Autodesk Inventor part; units mm, degrees
ref_plane "YZ Plane" through (0, 0, 0) normal (1, 0, 0) x (0, 1, 0)
ref_plane "XZ Plane" through (0, 0, 0) normal (0, 1, 0) x (-1, 0, 0)
ref_plane "XY Plane" through (0, 0, 0) normal (0, 0, 1) x (1, 0, 0)
sketch "Sketch1" plane through (0, 0, 0) normal (0, 1, 0) x (-1, 0, 0)
  line L0 (0, 0) -> (10, 0)
  line L1 (10, 0) -> (66.654, -9.9896)
  line L2 (66.654, -9.9896) -> (66.654, -41.5096)
  line L3 (66.654, -41.5096) -> (2, -133.8451)
  line L4 (2, -133.8451) -> (0, -133.8451)
  line L5 (0, -133.8451) -> (0, 0)
  dimension "d0" = 31.52
  dimension "d1" = 145
  dimension "d2" = 100
  dimension "d3" = 10
  dimension "d4" = 2
  dimension "d5" = 66.654
extrude "Extrusion1" add sketch "Sketch1" along normal blind 6.5
sketch "Sketch2" plane through (0, 6.5, 0) normal (0, 1, 0) x (1, 0, 0)
  line L0 (-66.654, 41.5096) -> (-66.654, 9.9896)
  line L1 (-66.654, 9.9896) -> (-10, 0)
  line L2 (-50.354, 26.3816) -> (-50.354, 21.8816)
  line L3 (-66.654, 21.8816) -> (-66.654, 26.3816)
  line L4 (-61.654, 28.8816) -> (-54.354, 28.8816)
  line L5 (-54.354, 19.3816) -> (-61.654, 19.3816)
  line L6 (-66.654, 26.3816) -> (-61.654, 26.3816)
  line L7 (-54.354, 26.3816) -> (-50.354, 26.3816)
  line L8 (-61.654, 19.3816) -> (-61.654, 21.8816)
  line L9 (-61.654, 26.3816) -> (-61.654, 28.8816)
  line L10 (-50.354, 21.8816) -> (-54.354, 21.8816)
  line L11 (-61.654, 21.8816) -> (-66.654, 21.8816)
  line L12 (-54.354, 28.8816) -> (-54.354, 26.3816)
  line L13 (-54.354, 21.8816) -> (-54.354, 19.3816)
  line L14 (-37.7124, 21.4379) -> (-33.2807, 20.6565)
  line L15 (-36.1112, 4.6041) -> (-40.5428, 5.3855)
  line L16 (-42.1366, 10.7437) -> (-40.869, 17.9328)
  line L17 (-31.5133, 16.2831) -> (-32.7809, 9.094)
  line L18 (-40.5428, 5.3855) -> (-39.6746, 10.3096)
  line L19 (-38.4069, 17.4987) -> (-37.7124, 21.4379)
  line L20 (-32.7809, 9.094) -> (-35.2429, 9.5281)
  line L21 (-39.6746, 10.3096) -> (-42.1366, 10.7437)
  line L22 (-33.2807, 20.6565) -> (-33.9753, 16.7172)
  line L23 (-35.2429, 9.5281) -> (-36.1112, 4.6041)
  line L24 (-40.869, 17.9328) -> (-38.4069, 17.4987)
  line L25 (-33.9753, 16.7172) -> (-31.5133, 16.2831)
  point P0 (-38.327, 4.9948)
  point P1 (-50.354, 24.1316)
  dimension "d8" = 4.5
  dimension "d9" = 5
  dimension "d10" = 4
  dimension "d11" = 7.3
  dimension "d12" = 2.5
  dimension "d13" = 4.5
  dimension "d14" = 5
  dimension "d15" = 4
  dimension "d16" = 7.3
  dimension "d17" = 2.5
  dimension "d35" = 14.142
extrude "Extrusion2" cut sketch "Sketch2" against normal through all
sketch "Sketch3" plane through (0, 6.5, 0) normal (0, 1, 0) x (1, 0, 0)
  line L0 (-66.654, 9.9896) -> (-40.5428, 5.3855)
  line L1 (-37.7124, 21.4379) -> (-33.2807, 20.6565)
  line L2 (-36.1112, 4.6041) -> (-10, 0)
  line L3 (-45.7131, 6.2972) -> (-53.5915, 7.6864)
  line L4 (-53.5915, 7.6864) -> (-54.3729, 3.2547)
  line L5 (-52.7506, 0.9378) -> (-48.8114, 0.2432)
  line L6 (-46.4945, 1.8655) -> (-45.7131, 6.2972)
  line L7 (-30.9409, 3.6925) -> (-23.0625, 2.3033)
  line L8 (-23.0625, 2.3033) -> (-23.8439, -2.1284)
  line L9 (-26.1608, -3.7507) -> (-30.1, -3.0561)
  line L10 (-31.7224, -0.7392) -> (-30.9409, 3.6925)
  arc A0 (-54.3729, 3.2547) -> (-52.7506, 0.9378) centre (-52.4033, 2.9074) ccw
  arc A1 (-48.8114, 0.2432) -> (-46.4945, 1.8655) centre (-48.4641, 2.2128) ccw
  arc A2 (-31.7224, -0.7392) -> (-30.1, -3.0561) centre (-29.7527, -1.0865) ccw
  arc A3 (-26.1608, -3.7507) -> (-23.8439, -2.1284) centre (-25.8135, -1.7811) ccw
  point P0 (-35.4965, 21.0472)
  dimension "d20" = 2
  dimension "d21" = 8
  dimension "d22" = 8
  dimension "d23" = 6.5
  dimension "d24" = 15
  dimension "d25" = 7.5
extrude "Extrusion3" add sketch "Sketch3" against normal blind 6.5
sketch "Sketch4" plane through (0, 6.5, 0) normal (0, 1, 0) x (1, 0, 0)
  line L0 (-23.0625, 2.3033) -> (-10, 0)
  line L1 (-10, 0) -> (0, 0)
  line L2 (0, 0) -> (0, 133.8451)
  line L3 (-61.654, 19.3816) -> (-61.654, 21.8816)
  line L4 (0, 50) -> (-10, 50)
  line L5 (-10, 50) -> (-14, 46)
  line L6 (-14, 46) -> (-14, 0.7053)
  dimension "d28" = 45
  dimension "d29" = 10
  dimension "d30" = 50
  dimension "d32" = 4
extrude "Extrusion4" cut sketch "Sketch4" against normal through all
sketch "Sketch5" plane through (0, 6.5, 0) normal (0, 1, 0) x (1, 0, 0)
  line L0 (0, 50) -> (0, 133.8451)
  line L1 (0, 62.001) -> (4.5, 62.001)
  line L2 (6.5, 64.001) -> (6.5, 68.001)
  line L3 (4.5, 70.001) -> (0, 70.001)
  line L4 (0, 70.001) -> (0, 62.001)
  arc A0 (4.5, 62.001) -> (6.5, 64.001) centre (4.5, 64.001) ccw
  arc A1 (6.5, 68.001) -> (4.5, 70.001) centre (4.5, 68.001) ccw
  point P0 (0, 0)
  dimension "d36" = 2
  dimension "d37" = 8
  dimension "d38" = 6.5
  dimension "d39" = 12.001
extrude "Extrusion5" add sketch "Sketch5" against normal blind 6.5
properties part number "front_panel_brace_middle" material "Plywood, Finish"
Here's how the part is built. I have some questions about the finished solid (model axes, mm). A direction names the side the tool comes from. Coordinates: 2 decimals unless noted, no trailing zeros. Order: outer loops, then holes, each group sorted by start corner. A loop starts at its lowest first (then second) coordinate and runs counter-clockwise, first axis right, second up. Notation, with made-up numbers: (-0.75, 7.25) - (3.25, 7.25) arc R12 ccw to (3.25, 12.25) - close; hole circle Ø1 at (73.25, 66). An arc over 180 degrees is marked (long way). Use CSV: the item, a comma, the result in double quotes. Start each with the question number.
1. Suppose I cut it at B-B on x = -11.5. List the corners of the cut face in (y, z) for me.
2. Suppose I cut it at A-A on z = -38.5. List the corners of the cut face in (x, y) for me, then the cut area to 3 significant figures.
3. Please list where these lines run through material, in increasing order: line 1 (X direction, y = 3, z = -2.5); line 2 (X direction, y = 2.25, z = -36); line 3 (X direction, y = 1.5, z = -7.5). Write a range as from..to.
4. If we mould it in two halves opening along Z, with no side actions, what happens to faces 5 (the face through (-12, 3, -48)), 6 (the face through (-52, 3, -26.382)), 7 (the face through (0, 3, -56))? For each: +Z half, -Z half, draft (parallel to the pull), parting line (faces both ways), or undercut.
5. I'm going to push flat-ended pins straight in: pin 1 (3.5 mm diameter, centred on x = 2.5, y = 3, fed in from -Z); pin 2 (3 mm diameter, centred on x = -7.5, y = 4, fed in from +Z); pin 3 (2 mm diameter, centred on y = 1, z = -17, fed in from +X). Where does each tip first touch, or does it pass through?
6. For faces 1 (the face through (-35.67, 3.3, -7.1)), 2 (the face through (-5, 3, -50)), 3 (the face through (-23.448, 3.296, -0.118)), 4 (the face through (-50.354, 3, -24)), which set-ups out of +Z, -Z, +X, -X, +Y, -Y let a thin tool reach every point of the face, with its end or its side?
Output:
1,outline,"(0, -120.28) - (6.5, -120.28) - (6.5, -48.5) - (0, -48.5) - close"
2,outline,"(-66.65, 0) - (-14, 0) - (-14, 6.5) - (-66.65, 6.5) - close"
2,area,"342 mm2"
3,line 1,"x = -54.36..-46.38, -31.15..-14"
3,line 2,"x = -66.65..-14"
3,line 3,"x = -53.62..-40.17, -35.6..-14"
4,face 5,"+Z half"
4,face 6,"undercut"
4,face 7,"draft"
5,pin 1,"stops at z = -70"
5,pin 2,"stops at z = -50"
5,pin 3,"stops at x = -14"
6,face 1,"+Y, -Y"
6,face 2,"+Z, +X, +Y, -Y"
6,face 3,"+Z, +Y, -Y"
6,face 4,"-X, +Y, -Y"
